The listing builds one solid part. Answer for the finished solid, in the listing's coordinates (mm). Coordinates: 2 decimals unless noted, no trailing zeros. Order: outer loops, then holes, each group sorted by start corner. A loop starts at its lowest first (then second) coordinate and runs counter-clockwise, first axis right, second up. Notation, with made-up numbers: (41, -35) -> (91, -35) arc R15 cw to (91, -14) -> close; hole circle Ø4 at (89.25, -16.5). An arc over 180 degrees is marked (long way). Answer in a Markdown table with one row per item. Add a question column.
```python
from build123d import *

# Parameters (mm, degrees)
EXTRUDE1_DEPTH                                = 25.4
FILLET1_R                                     = 25.4
CHAMFER1_SIZE                                 = 1.524
CBORE_FOR_3_8_SOCKET_HEAD_CAP_SCREW1_AT_COUNT = 2
CBORE_FOR_3_8_SOCKET_HEAD_CAP_SCREW1_AT_PITCH = 76.2
CBORE_FOR_3_8_SOCKET_HEAD_CAP_SCREW1_2_COUNT  = 2
CBORE_FOR_3_8_SOCKET_HEAD_CAP_SCREW1_2_PITCH  = 76.2
CBORE_FOR_3_8_SOCKET_HEAD_CAP_SCREW1_3_COUNT  = 2
CBORE_FOR_3_8_SOCKET_HEAD_CAP_SCREW1_3_PITCH  = 152.4
CIRPATTERN1_COUNT                             = 6


with BuildPart() as part:
    # Sketch1 → Extrude1 (new body)
    with BuildSketch(Plane.XY):
        Polygon((169.560557183, 293.6875), (-169.560557183, 293.6875), (-339.121114365, 0), (-169.560557183, -293.6875), (169.560557183, -293.6875), (339.121114365, 0), align=None)
    extrude(amount=EXTRUDE1_DEPTH)

    # Fillet1
    fillet1_edges = [part.edges().sort_by_distance(p)[0] for p in [
        (-169.560557183, -293.6875, 12.7),
        (-339.121114365, 0, 12.7),
        (-169.560557183, 293.6875, 12.7),
        (169.560557183, 293.6875, 12.7),
        (339.121114365, 0, 12.7),
        (169.560557183, -293.6875, 12.7),
    ]]
    fillet(fillet1_edges, radius=FILLET1_R)

    # Chamfer1
    chamfer1_edges = [part.edges().sort_by_distance(p)[0] for p in [
        (-254.340835774, -146.84375, 0),
        (-254.340835774, -146.84375, 25.4),
        (254.340835774, 146.84375, 0),
        (254.340835774, -146.84375, 0),
        (0, -293.6875, 0),
        (-254.340835774, 146.84375, 0),
        (0, 293.6875, 0),
        (167.595860345, 290.284545256, 0),
        (-167.595860345, 290.284545256, 0),
        (335.19172069, 0, 0),
        (167.595860345, -290.284545256, 0),
        (-167.595860345, -290.284545256, 0),
        (-335.19172069, 0, 0),
        (-254.340835774, 146.84375, 25.4),
        (254.340835774, 146.84375, 25.4),
        (0, 293.6875, 25.4),
        (0, -293.6875, 25.4),
        (254.340835774, -146.84375, 25.4),
        (167.595860345, 290.284545256, 25.4),
        (-167.595860345, 290.284545256, 25.4),
        (335.19172069, 0, 25.4),
        (167.595860345, -290.284545256, 25.4),
        (-167.595860345, -290.284545256, 25.4),
        (-335.19172069, 0, 25.4),
    ]]
    chamfer(chamfer1_edges, length=CHAMFER1_SIZE)

    # Sketch2 → CBORE for 3_8 Socket Head Cap Screw1 (revolve, cut)
    with BuildSketch(Plane(origin=(-38.1, -282.575, 25.4), x_dir=(0, -1, 0), z_dir=(1, 0, 0))):
        Polygon((0, 0), (0, 25.4), (5.842, 25.4), (5.15874, 24.613999282), (5.15874, 10.668), (8.7376, 10.668), (8.7376, 0), align=None)
    cbore_for_3_8_socket_head_cap_screw1 = revolve(axis=Axis((-38.1, -282.575, 31.75), (0, 0, -1)), mode=Mode.SUBTRACT)

    # CBORE for 3_8 Socket Head Cap Screw1 at: CBORE for 3_8 Socket Head Cap Screw1 ×2
    with Locations(*[(-i * CBORE_FOR_3_8_SOCKET_HEAD_CAP_SCREW1_AT_PITCH, 0, 0) for i in range(1, CBORE_FOR_3_8_SOCKET_HEAD_CAP_SCREW1_AT_COUNT)]):
        add(cbore_for_3_8_socket_head_cap_screw1, mode=Mode.SUBTRACT)

    # CBORE for 3_8 Socket Head Cap Screw1 2: CBORE for 3_8 Socket Head Cap Screw1 ×2
    with Locations(*[(i * CBORE_FOR_3_8_SOCKET_HEAD_CAP_SCREW1_2_PITCH, 0, 0) for i in range(1, CBORE_FOR_3_8_SOCKET_HEAD_CAP_SCREW1_2_COUNT)]):
        add(cbore_for_3_8_socket_head_cap_screw1, mode=Mode.SUBTRACT)

    # CBORE for 3_8 Socket Head Cap Screw1 3: CBORE for 3_8 Socket Head Cap Screw1 ×2
    with Locations(*[(i * CBORE_FOR_3_8_SOCKET_HEAD_CAP_SCREW1_3_PITCH, 0, 0) for i in range(1, CBORE_FOR_3_8_SOCKET_HEAD_CAP_SCREW1_3_COUNT)]):
        add(cbore_for_3_8_socket_head_cap_screw1, mode=Mode.SUBTRACT)

    # CirPattern1: CBORE for 3_8 Socket Head Cap Screw1 ×6 about axis
    cirpattern1_axis = Axis((0, 0, 0), (0, 0, 1))
    for i in range(1, CIRPATTERN1_COUNT):
        add(cbore_for_3_8_socket_head_cap_screw1.rotate(cirpattern1_axis, i * 360 / CIRPATTERN1_COUNT), mode=Mode.SUBTRACT)

    # CirPattern1 copy 1 sketch → CirPattern1 copy 1 (revolve, cut)
    with BuildSketch(Plane(origin=(187.567128474, -240.274203653, 25.4), x_dir=(0.866025404, -0.5, 0), z_dir=(0.5, 0.866025404, 0))):
        Polygon((0, 0), (0, 25.4), (5.842, 25.4), (5.15874, 24.613999282), (5.15874, 10.668), (8.7376, 10.668), (8.7376, 0), align=None)
    revolve(axis=Axis((187.567128474, -240.274203653, 31.75), (0, 0, -1)), mode=Mode.SUBTRACT)

    # CirPattern1 copy 2 sketch → CirPattern1 copy 2 (revolve, cut)
    with BuildSketch(Plane(origin=(301.867128474, 42.300796347, 25.4), x_dir=(0.866025404, 0.5, 0), z_dir=(-0.5, 0.866025404, 0))):
        Polygon((0, 0), (0, 25.4), (5.842, 25.4), (5.15874, 24.613999282), (5.15874, 10.668), (8.7376, 10.668), (8.7376, 0), align=None)
    revolve(axis=Axis((301.867128474, 42.300796347, 31.75), (0, 0, -1)), mode=Mode.SUBTRACT)

    # CirPattern1 copy 3 sketch → CirPattern1 copy 3 (revolve, cut)
    with BuildSketch(Plane(origin=(114.3, 282.575, 25.4), x_dir=(0, 1, 0), z_dir=(-1, 0, 0))):
        Polygon((0, 0), (0, 25.4), (5.842, 25.4), (5.15874, 24.613999282), (5.15874, 10.668), (8.7376, 10.668), (8.7376, 0), align=None)
    revolve(axis=Axis((114.3, 282.575, 31.75), (0, 0, -1)), mode=Mode.SUBTRACT)

    # CirPattern1 copy 4 sketch → CirPattern1 copy 4 (revolve, cut)
    with BuildSketch(Plane(origin=(-187.567128474, 240.274203653, 25.4), x_dir=(-0.866025404, 0.5, 0), z_dir=(-0.5, -0.866025404, 0))):
        Polygon((0, 0), (0, 25.4), (5.842, 25.4), (5.15874, 24.613999282), (5.15874, 10.668), (8.7376, 10.668), (8.7376, 0), align=None)
    revolve(axis=Axis((-187.567128474, 240.274203653, 31.75), (0, 0, -1)), mode=Mode.SUBTRACT)

    # CirPattern1 copy 5 sketch → CirPattern1 copy 5 (revolve, cut)
    with BuildSketch(Plane(origin=(-301.867128474, -42.300796347, 25.4), x_dir=(-0.866025404, -0.5, 0), z_dir=(0.5, -0.866025404, 0))):
        Polygon((0, 0), (0, 25.4), (5.842, 25.4), (5.15874, 24.613999282), (5.15874, 10.668), (8.7376, 10.668), (8.7376, 0), align=None)
    revolve(axis=Axis((-301.867128474, -42.300796347, 31.75), (0, 0, -1)), mode=Mode.SUBTRACT)

    # CirPattern1 copy 6 sketch → CirPattern1 copy 6 (revolve, cut)
    with BuildSketch(Plane(origin=(263.767128474, -108.291932116, 25.4), x_dir=(0.866025404, -0.5, 0), z_dir=(0.5, 0.866025404, 0))):
        Polygon((0, 0), (0, 25.4), (5.842, 25.4), (5.15874, 24.613999282), (5.15874, 10.668), (8.7376, 10.668), (8.7376, 0), align=None)
    revolve(axis=Axis((263.767128474, -108.291932116, 31.75), (0, 0, -1)), mode=Mode.SUBTRACT)

    # CirPattern1 copy 7 sketch → CirPattern1 copy 7 (revolve, cut)
    with BuildSketch(Plane(origin=(225.667128474, 174.283067884, 25.4), x_dir=(0.866025404, 0.5, 0), z_dir=(-0.5, 0.866025404, 0))):
        Polygon((0, 0), (0, 25.4), (5.842, 25.4), (5.15874, 24.613999282), (5.15874, 10.668), (8.7376, 10.668), (8.7376, 0), align=None)
    revolve(axis=Axis((225.667128474, 174.283067884, 31.75), (0, 0, -1)), mode=Mode.SUBTRACT)

    # CirPattern1 copy 8 sketch → CirPattern1 copy 8 (revolve, cut)
    with BuildSketch(Plane(origin=(-38.1, 282.575, 25.4), x_dir=(0, 1, 0), z_dir=(-1, 0, 0))):
        Polygon((0, 0), (0, 25.4), (5.842, 25.4), (5.15874, 24.613999282), (5.15874, 10.668), (8.7376, 10.668), (8.7376, 0), align=None)
    revolve(axis=Axis((-38.1, 282.575, 31.75), (0, 0, -1)), mode=Mode.SUBTRACT)

    # CirPattern1 copy 9 sketch → CirPattern1 copy 9 (revolve, cut)
    with BuildSketch(Plane(origin=(-263.767128474, 108.291932116, 25.4), x_dir=(-0.866025404, 0.5, 0), z_dir=(-0.5, -0.866025404, 0))):
        Polygon((0, 0), (0, 25.4), (5.842, 25.4), (5.15874, 24.613999282), (5.15874, 10.668), (8.7376, 10.668), (8.7376, 0), align=None)
    revolve(axis=Axis((-263.767128474, 108.291932116, 31.75), (0, 0, -1)), mode=Mode.SUBTRACT)

    # CirPattern1 copy 10 sketch → CirPattern1 copy 10 (revolve, cut)
    with BuildSketch(Plane(origin=(-225.667128474, -174.283067884, 25.4), x_dir=(-0.866025404, -0.5, 0), z_dir=(0.5, -0.866025404, 0))):
        Polygon((0, 0), (0, 25.4), (5.842, 25.4), (5.15874, 24.613999282), (5.15874, 10.668), (8.7376, 10.668), (8.7376, 0), align=None)
    revolve(axis=Axis((-225.667128474, -174.283067884, 31.75), (0, 0, -1)), mode=Mode.SUBTRACT)

    # CirPattern1 copy 11 sketch → CirPattern1 copy 11 (revolve, cut)
    with BuildSketch(Plane(origin=(301.867128474, -42.300796347, 25.4), x_dir=(0.866025404, -0.5, 0), z_dir=(0.5, 0.866025404, 0))):
        Polygon((0, 0), (0, 25.4), (5.842, 25.4), (5.15874, 24.613999282), (5.15874, 10.668), (8.7376, 10.668), (8.7376, 0), align=None)
    revolve(axis=Axis((301.867128474, -42.300796347, 31.75), (0, 0, -1)), mode=Mode.SUBTRACT)

    # CirPattern1 copy 12 sketch → CirPattern1 copy 12 (revolve, cut)
    with BuildSketch(Plane(origin=(187.567128474, 240.274203653, 25.4), x_dir=(0.866025404, 0.5, 0), z_dir=(-0.5, 0.866025404, 0))):
        Polygon((0, 0), (0, 25.4), (5.842, 25.4), (5.15874, 24.613999282), (5.15874, 10.668), (8.7376, 10.668), (8.7376, 0), align=None)
    revolve(axis=Axis((187.567128474, 240.274203653, 31.75), (0, 0, -1)), mode=Mode.SUBTRACT)

    # CirPattern1 copy 13 sketch → CirPattern1 copy 13 (revolve, cut)
    with BuildSketch(Plane(origin=(-114.3, 282.575, 25.4), x_dir=(0, 1, 0), z_dir=(-1, 0, 0))):
        Polygon((0, 0), (0, 25.4), (5.842, 25.4), (5.15874, 24.613999282), (5.15874, 10.668), (8.7376, 10.668), (8.7376, 0), align=None)
    revolve(axis=Axis((-114.3, 282.575, 31.75), (0, 0, -1)), mode=Mode.SUBTRACT)

    # CirPattern1 copy 14 sketch → CirPattern1 copy 14 (revolve, cut)
    with BuildSketch(Plane(origin=(-301.867128474, 42.300796347, 25.4), x_dir=(-0.866025404, 0.5, 0), z_dir=(-0.5, -0.866025404, 0))):
        Polygon((0, 0), (0, 25.4), (5.842, 25.4), (5.15874, 24.613999282), (5.15874, 10.668), (8.7376, 10.668), (8.7376, 0), align=None)
    revolve(axis=Axis((-301.867128474, 42.300796347, 31.75), (0, 0, -1)), mode=Mode.SUBTRACT)

    # CirPattern1 copy 15 sketch → CirPattern1 copy 15 (revolve, cut)
    with BuildSketch(Plane(origin=(-187.567128474, -240.274203653, 25.4), x_dir=(-0.866025404, -0.5, 0), z_dir=(0.5, -0.866025404, 0))):
        Polygon((0, 0), (0, 25.4), (5.842, 25.4), (5.15874, 24.613999282), (5.15874, 10.668), (8.7376, 10.668), (8.7376, 0), align=None)
    revolve(axis=Axis((-187.567128474, -240.274203653, 31.75), (0, 0, -1)), mode=Mode.SUBTRACT)


solid = part.part
```
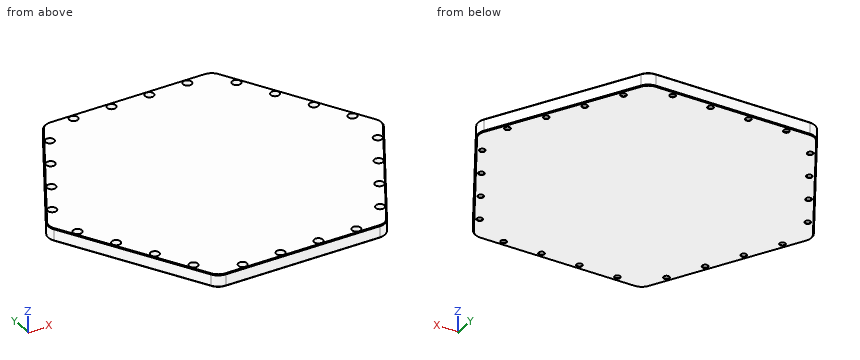
Q1. A cutting plane is placed at B-B (x = 204.5). Determine the outline of the cut face in (y, z), then the cut area to 3 significant figures.
Q2. A cutting plane is placed at C-C (z = 5.5). State how many separate pieces and enclosed holes the cut face has, then the cut area to 3 significant figures.
Q3. Straight lines are drawn through the part: line 1 (Y direction, x = -187, z = 3.25); line 2 (Y direction, x = -298, z = 21.25); line 3 (X direction, y = -13, z = 7). For each, find the intervals that lie inside material, in ascending order.
Q4. Given pin 1 (10.5 mm diameter, centred on x = -187.57, y = 240.27, fed in from +Z); pin 2 (4 mm diameter, centred on x = 217.5, z = 14, fed in from +Y); pin 3 (3 mm diameter, centred on y = 188.5, z = 8, fed in from +X), each flat-ended and moving along its own axis, determine where each tip first touches the part or whether it passes through.
Q5. A cutting plane is placed at A-A (y = 130.5). Determine the outline of the cut face in (x, z).
Returned:
| question | item | result |
|---|---|---|
| 1 | outline | (-233.17, 1.52) -> (-230.12, 0) -> (230.12, 0) -> (233.17, 1.52) -> (233.17, 23.88) -> (230.12, 25.4) -> (-230.12, 25.4) -> (-233.17, 23.88) -> close |
| 1 | area | 11,800 mm² |
| 2 | separate pieces | 1 |
| 2 | enclosed holes | 24 |
| 2 | area | 297,000 mm² |
| 3 | line 1 | y = -263.48 to -245.4, -235.15 to 235.15, 245.4 to 263.48 |
| 3 | line 2 | y = -71.22 to -50.14, -34.47 to 34.47, 50.14 to 71.22 |
| 3 | line 3 | x = -331.62 to 331.62 |
| 4 | pin 1 | stops at z = 14.73 |
| 4 | pin 2 | stops at y = 214.12 |
| 4 | pin 3 | stops at x = 231.16 |
| 5 | outline | (-263.78, 1.52) -> (-262.02, 0) -> (262.02, 0) -> (263.78, 1.52) -> (263.78, 23.88) -> (262.02, 25.4) -> (-262.02, 25.4) -> (-263.78, 23.88) -> close |
